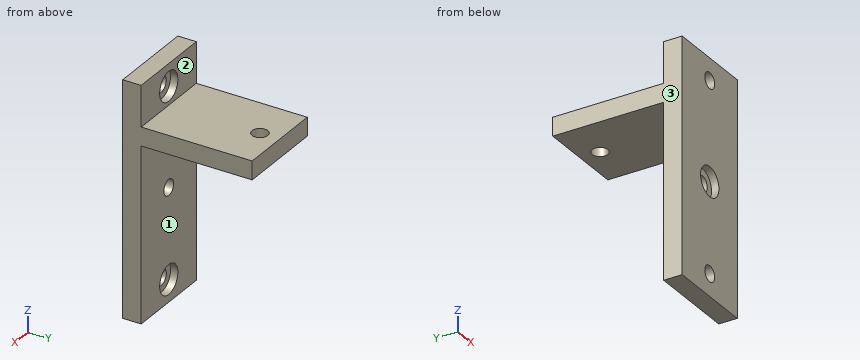
Autodesk Inventor part; units mm, degrees
ref_plane "YZ Plane" through (0, 0, 0) normal (1, 0, 0) x (0, 1, 0)
ref_plane "XZ Plane" through (0, 0, 0) normal (0, 1, 0) x (-1, 0, 0)
ref_plane "XY Plane" through (0, 0, 0) normal (0, 0, 1) x (1, 0, 0)
sketch "Sketch14" plane through (0, 0, 0) normal (0, 1, 0) x (-1, 0, 0)
  line L0 (12, 14) -> (-12, 14)
  line L1 (-12, 14) -> (-12, -14)
  line L2 (-12, -14) -> (12, -14)
  line L3 (12, -14) -> (12, 14)
  line L4 (12, 14) -> (-12, -14) construction
  line L5 (-12, 14) -> (12, -14) construction
  line L6 (12, 14) -> (-12, 14)
  line L7 (-12, 14) -> (-12, 30)
  line L8 (-12, 30) -> (12, 30)
  line L9 (12, 30) -> (12, 14)
  line L10 (-12, -14) -> (12, -14)
  line L11 (12, -14) -> (12, -33)
  line L12 (12, -33) -> (-12, -33)
  line L13 (-12, -33) -> (-12, -14)
  point P0 (0, 0)
  point P1 (12, -14)
  dimension "d93" = 28
  dimension "d94" = 24
  dimension "d95" = 16
  dimension "d111" = 19
extrude "Extrusion8" add sketch "Sketch14" along normal blind 5
sketch "Sketch17" plane through (0, 5, 0) normal (0, 1, 0) x (1, 0, 0)
  line L0 (-12, -30) -> (12, -30)
  line L1 (12, 33) -> (-12, 33)
  point P0 (0, 0)
  point P1 (0, 27)
  point P2 (0, -24)
  dimension "d119" = 0
  dimension "d121" = 6
  dimension "d122" = 0
  dimension "d125" = 6
hole "Hole8" at (0, 5, -27) at (0, 5, 24) direction (0, -1, 0) diameter 4.305 end through all counterbore diameter 7.938 counterbore depth 2
sketch "Sketch18" plane through (0, 5, 0) normal (0, 1, 0) x (1, 0, 0)
  line L0 (12, -30) -> (12, 33)
  line L1 (-12, 33) -> (-12, -30)
  line L2 (12, -14) -> (-12, -14)
  line L3 (-12, -14) -> (-12, -19)
  line L4 (-12, -19) -> (12, -19)
  line L5 (12, -19) -> (12, -14)
  point P0 (0, 0)
  point P1 (-12, -14)
  dimension "d126" = 5
  dimension "d127" = 14
extrude "Extrusion10" add sketch "Sketch18" along normal blind 30
sketch "Sketch19" plane through (-12, 5, 19) normal (0, 0, 1) x (1, 0, 0)
  line L0 (0, 0) -> (24, 0)
  line L1 (0, 0) -> (0, 30)
  point P0 (12, -5)
  point P1 (12, 24.659)
  dimension "d138" = 24.659
  dimension "d148" = 12
hole "Hole9" at (0, 29.659, 19) direction (0, 0, -1) diameter 4.3 depth 11.8
sketch "Sketch20" plane through (0, 0, 0) normal (0, -1, 0) x (1, 0, 0)
  line L0 (-12, 14) -> (12, 14)
  point P0 (0, 0)
  point P1 (0, -2.678)
  dimension "d146" = 16.678
  dimension "d147" = 0
hole "Hole10" at (0, 0, -2.678) direction (0, 1, 0) diameter 4.3 depth 11.8 counterbore diameter 8 counterbore depth 2
equation "\"LASER_HOLE_HEIGHT\" = 16.7"
equation "\"a\" = 24.659"
equation "\"b\" = 16.678"
properties part number "UEOM L mount Vertical"
Model file for the job. Use its own axes, mm. Face numbers are marked on the shaded views. A direction names the side the tool comes from. Round coordinates to 2 decimals unless told otherwise and drop trailing zeros. Write each loop counter-clockwise with the first axis right and the second up, starting at its lowest first coordinate (ties: lowest second). Pieces come first, ordered by that corner, then holes. Notation, with made-up numbers: (34, 53) -> (86, 53) arc R19 ccw to (86, 57) -> close; hole circle Ø4 at (69, 35.5). An arc over 180 degrees is marked (long way). Answer as CSV lines item,"result".
1. Slice it at B-B, the plane x = 5.5. List the corners of the cut face in (y, z), plus the area to 3 significant figures.
Resolved:
outline,"(0, -33) -> (5, -33) -> (5, 14) -> (35, 14) -> (35, 19) -> (5, 19) -> (5, 30) -> (0, 30) -> close"
area,"465 mm²"
2. Tool access for the marked faces 1, 2 and 3: list every direction of +Z, -Z, +X, -X, +Y, -Y with a clear straight run to the whole face (end or side of a thin tool).
Resolved:
face 1,"-Z, +X, -X, +Y"
face 2,"+Z, +X, -X, +Y"
face 3,"+Z, -Z, -X, +Y, -Y"
3. Pin check, flat tips, straight feed: pin 1 Ø3.5 at (x, z) = (3.5, 22.5) entering from +Y; pin 2 Ø2 at (x, y) = (-7.5, 22.5) entering from -Z; pin 3 Ø5 at (x, y) = (-7.5, 14.5) entering from +Z. Stop position of each tip, or through.
Resolved:
pin 1,"y = 5"
pin 2,"z = 14"
pin 3,"z = 19"
4. Slice it at D-D, the plane z = -5.5. List the corners of the cut face in (x, y).
Resolved:
outline,"(-12, 0) -> (-2.83, 0) -> (-2.83, 2) -> (2.83, 2) -> (2.83, 0) -> (12, 0) -> (12, 5) -> (-12, 5) -> close"
5. Slice it at C-C, the plane x = 0. State how many separate pieces and enclosed holes the cut face has, plus the area to 3 significant figures.
Resolved:
separate pieces,"5"
enclosed holes,"0"
area,"357 mm²"
6. Drill centre lines: line 1 (Z direction, x = 0, y = 0.7); line 2 (Z direction, x = 0, y = 3.9); line 3 (X direction, y = 3.85, z = -27). Where is each one in solid material? Low to high.
Resolved:
line 1,"-33 to -29.15, -24.85 to -6.68, 1.32 to 21.85, 26.15 to 30"
line 2,"-33 to -30.97, -23.03 to -4.83, -0.53 to 20.03, 27.97 to 30"
line 3,"-12 to -3.97, 3.97 to 12"
7. Slice it at A-A, the plane z = -27. List the corners of the cut face in (x, y).
Resolved:
outline,"(-12, 0) -> (-2.15, 0) -> (-2.15, 3) -> (-3.97, 3) -> (-3.97, 5) -> (-12, 5) -> close; (2.15, 0) -> (12, 0) -> (12, 5) -> (3.97, 5) -> (3.97, 3) -> (2.15, 3) -> close"
